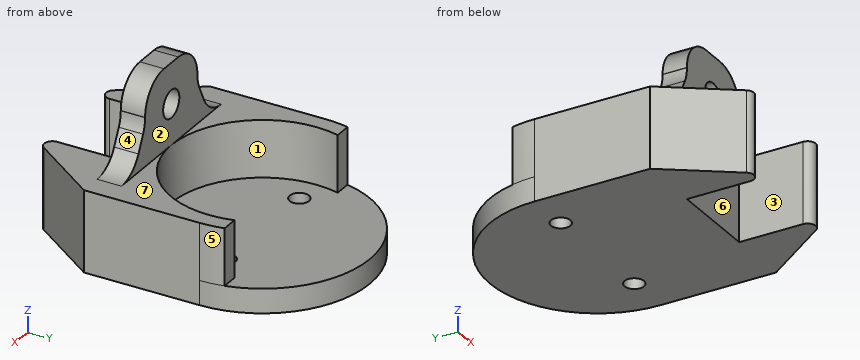
```python
from build123d import *

# Parameters (mm, degrees)
PAD_DEPTH    = 3
PAD001_DEPTH = 7
SKETCH001_R  = 1.2
POCKET_DEPTH = 3.001
SKETCH003_R  = 1.7
PAD002_DEPTH = 3
FILLET_R     = 4
FILLET001_R  = 1


with BuildPart() as part:
    # Sketch → Pad (new body)
    with BuildSketch(Plane.XY):
        with BuildLine():
            Line((5.5, -14.25), (5.5, -25.25))
            Line((5.5, -25.25), (13.25, -14.25))
            Line((13.25, -14.25), (13.25, 0))
            ThreePointArc((13.25, 0), (0, 13.25), (-13.25, 0))
            Line((-13.25, -14.25), (-13.25, 0))
            Line((-13.25, -14.25), (-5.5, -25.25))
            Line((-5.5, -25.25), (-5.5, -14.25))
            Line((-5.5, -14.25), (5.5, -14.25))
        make_face()
    extrude(amount=PAD_DEPTH)

    # Sketch002 → Pad001 (join)
    with BuildSketch(Plane.XY.offset(3)):
        with BuildLine():
            Line((-13.25, 0), (-13.25, -14.25))
            Line((-13.25, -14.25), (-5.5, -25.25))
            Line((-5.5, -25.25), (-5.5, -14.25))
            Line((-5.5, -14.25), (5.5, -14.25))
            Line((5.5, -14.25), (5.5, -25.25))
            Line((5.5, -25.25), (13.25, -14.25))
            Line((13.25, -14.25), (13.25, 0))
            ThreePointArc((13.25, 0), (13.169004, 1.462815), (12.927007, 2.907747))
            Line((10.867728, 2.907747), (12.927007, 2.907747))
            ThreePointArc((-10.867728, 2.907747), (0, -11.25), (10.867728, 2.907747))
            Line((-12.927007, 2.907747), (-10.867728, 2.907747))
            ThreePointArc((-12.927007, 2.907747), (-13.169004, 1.462815), (-13.25, 0))
        make_face()
    extrude(amount=PAD001_DEPTH)

    # Sketch001 (on Face10 of Pad) → Pocket (cut, through all)
    with BuildSketch(Plane.XY.offset(3)):
        with Locations((-7.75, 0)):
            Circle(SKETCH001_R)
        with Locations((7.75, 0)):
            Circle(SKETCH001_R)
    extrude(amount=-POCKET_DEPTH, mode=Mode.SUBTRACT)

    # Sketch003 (on Face19 of Pocket) → Pad002 (join)
    with BuildSketch(Plane.XZ.offset(14.25)):
        Polygon((-5.5, 15), (-8, 10), (8, 10), (5.5, 15), (5.5, 20), (-5.5, 20), align=None)
        with Locations((0, 15)):
            Circle(SKETCH003_R, mode=Mode.SUBTRACT)
    extrude(amount=-PAD002_DEPTH)

    # Fillet
    fillet_edges = [part.edges().sort_by_distance(p)[0] for p in [
        (-5.5, -12.75, 15),
        (-5.5, -12.75, 20),
        (-8, -12.75, 10),
        (8, -12.75, 10),
        (5.5, -12.75, 15),
        (5.5, -12.75, 20),
    ]]
    fillet(fillet_edges, radius=FILLET_R)

    # Fillet001
    fillet001_edges = [part.edges().sort_by_distance(p)[0] for p in [
        (5.5, -25.25, 6.5),
        (5.5, -25.25, 1.5),
        (-5.5, -25.25, 6.5),
        (-5.5, -25.25, 1.5),
    ]]
    fillet(fillet001_edges, radius=FILLET001_R)


solid = part.part
```
Input: part model. Units: mm. Frame: model coordinates. Face numbers are marked on the shaded views. A direction names the side the tool comes from. Give positions to 0.01 mm unless a question says otherwise; leave off trailing zeros. Order: outer loops, then holes, each group sorted by start corner. A loop starts at its lowest first (then second) coordinate and runs counter-clockwise, first axis right, second up. Notation, with made-up numbers: M 17.5,31 L 30.5,31 A23 ccw 30.5,42 Z; hole C 30.25,42 d3. An arc over 180 degrees is marked long. Return JSON: item names as keys, results as strings.
1) Section query A-A on y = -17. Output: boundary loops of the cut face in (x, z), and give its area (3 significant figures).
Taken from the geometry:
{"outline": "M -11.31,0 L -5.5,0 L -5.5,10 L -11.31,10 Z; M 5.5,0 L 11.31,0 L 11.31,10 L 5.5,10 Z", "area": "116 mm2"}
2) Section query C-C on z = 2.5. Output: boundary loops of the cut face in (x, y), and give its area (3 significant figures).
Taken from the geometry:
{"outline": "M -13.25,-14.25 L -7.32,-22.67 A1 ccw -5.5,-22.09 L -5.5,-14.25 L 5.5,-14.25 L 5.5,-22.09 A1 ccw 7.32,-22.67 L 13.25,-14.25 L 13.25,0 A13.25 ccw -13.25,0 Z; hole C -7.75,0 d2.4; hole C 7.75,0 d2.4", "area": "726 mm2"}
3) Access query for the marked faces 1, 2, 3 and 4. Directions: +Z, -Z, +X, -X, +Y, -Y. A direction counts if a zero-diameter tool reaches every point of the face in a straight line with its end or side. Return the directions, or none.
Taken from the geometry:
{"face 1": "+Z", "face 2": "+Z, +X, -X, +Y", "face 3": "+Z, -Z, -Y", "face 4": "+Z, +X, +Y, -Y"}
4) Line query: L1, parallel to X at y = 0, z = 4.5; L2, parallel to Z at x = 0, y = -12.35; L3, parallel to Y at x = 7.75, z = 1.3. Output: solid intervals per line, ascending. Write a range as [from, to].
Taken from the geometry:
{"L1": "x = [-13.25, -11.25], [11.25, 13.25]", "L2": "z = [0, 13.3], [16.7, 20]", "L3": "y = [-22.06, -1.2], [1.2, 10.75]"}
5) Section query B-B on x = 7.75. Output: boundary loops of the cut face in (y, z), and give its area (3 significant figures).
Taken from the geometry:
{"outline": "M -22.06,0 L -1.2,0 L -1.2,3 L -8.15,3 L -8.15,10 L -11.25,10 L -11.25,11.07 L -14.25,11.07 L -14.25,10 L -22.06,10 Z; M 1.2,0 L 10.75,0 L 10.75,3 L 1.2,3 Z", "area": "192 mm2"}
6) Section query D-D on z = 5.5. Output: boundary loops of the cut face in (x, y).
Taken from the geometry:
{"outline": "M -13.25,-14.25 L -7.32,-22.67 A1 ccw -5.5,-22.09 L -5.5,-14.25 L 5.5,-14.25 L 5.5,-22.09 A1 ccw 7.32,-22.67 L 13.25,-14.25 L 13.25,0 A13.25 ccw 12.93,2.91 L 10.87,2.91 A11.25 cw long -10.87,2.91 L -12.93,2.91 A13.25 ccw -13.25,0 Z"}
7) Mould query, pull axis X, two halves, no side actions, for the marked faces 5, 6 and 7. Classes: released by +X, released by -X, zero draft, split by the parting line, or undercut.
Taken from the geometry:
{"face 5": "released by +X", "face 6": "undercut", "face 7": "zero draft"}
8) Contact query for flat-ended pins moving along their axis: pin 1 (8 mm diameter, centred on x = -8, y = 4, fed in from +Z); pin 2 (1.9 mm diameter, centred on x = -7.75, y = 0, fed in from +Z); pin 3 (3 mm diameter, centred on x = -4, z = 13, fed in from +Y); pin 4 (10.5 mm diameter, centred on x = -8, y = -8.5, fed in from +Z). Output: stop coordinate, or through.
Taken from the geometry:
{"pin 1": "stops at z = 10", "pin 2": "passes through", "pin 3": "stops at y = -11.25", "pin 4": "stops at z = 19.45"}
